Check sheet for the modelled part. Datum: model origin and axes. Units: mm. Face numbers are marked on the shaded views. A direction names the side the tool comes from. Give positions to 0.01 mm unless a question says otherwise; leave off trailing zeros. Order: outer loops, then holes, each group sorted by start corner. A loop starts at its lowest first (then second) coordinate and runs counter-clockwise, first axis right, second up.
from build123d import *

# Parameters (mm, degrees)
SKETCH_1_R      = 3.5
SKETCH_1_R_2    = 1.4
EXTRUDE_1_DEPTH = 2


with BuildPart() as part:
    # 草图1 → 凸台-拉伸1 (new body)
    with BuildSketch(Plane.XY):
        with BuildLine():
            Line((-10, -2), (-6.34428877, -2))
            ThreePointArc((-6.34428877, -2), (-5.378196987, -2.248809928), (-4.652478431, -2.933333333))
            ThreePointArc((-4.652478431, -2.933333333), (0, -5.5), (4.652478431, -2.933333333))
            ThreePointArc((4.652478431, -2.933333333), (5.378196987, -2.248809928), (6.34428877, -2))
            Line((6.34428877, -2), (10, -2))
            Line((10, -2), (10, 2))
            Line((10, 2), (6.34428877, 2))
            ThreePointArc((6.34428877, 2), (5.378196987, 2.248809928), (4.652478431, 2.933333333))
            ThreePointArc((4.652478431, 2.933333333), (0, 5.5), (-4.652478431, 2.933333333))
            ThreePointArc((-4.652478431, 2.933333333), (-5.378196987, 2.248809928), (-6.34428877, 2))
            Line((-6.34428877, 2), (-10, 2))
            Line((-10, 2), (-10, -2))
        make_face()
        Circle(SKETCH_1_R, mode=Mode.SUBTRACT)
        with Locations((-7.5, 0)):
            Circle(SKETCH_1_R_2, mode=Mode.SUBTRACT)
        with Locations((7.5, 0)):
            Circle(SKETCH_1_R_2, mode=Mode.SUBTRACT)
    extrude(amount=EXTRUDE_1_DEPTH)


solid = part.part
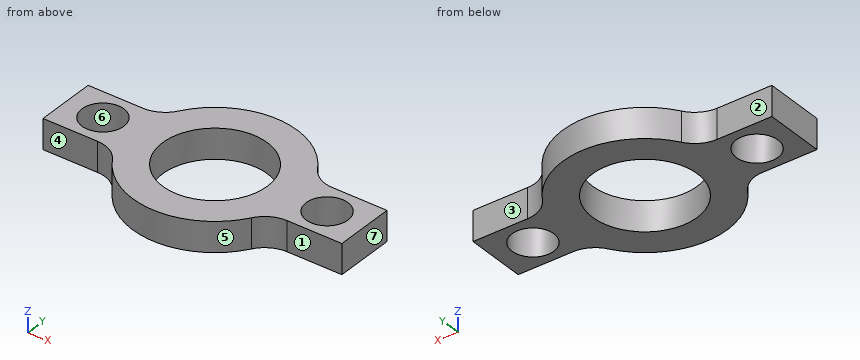
1) Draft check along X on the marked faces 5, 6 and 7. Enter one of: +X half, -X half, draft (parallel to the pull), parting line (faces both ways), or undercut.
Recorded:
face 5: parting line
face 6: undercut
face 7: +X half
2) Section check A-A, the plane y = 0. Record the cut outline in (x, z), then the cut area to 3 significant figures.
Recorded:
outline: (-10, 0) - (-8.9, 0) - (-8.9, 2) - (-10, 2) - close; (-6.1, 0) - (-3.5, 0) - (-3.5, 2) - (-6.1, 2) - close; (3.5, 0) - (6.1, 0) - (6.1, 2) - (3.5, 2) - close; (8.9, 0) - (10, 0) - (10, 2) - (8.9, 2) - close
area: 14.8 mm2
3) Section check C-C, the plane z = 1.45. Record the cut outline in (x, y), then the cut area to 3 significant figures.
Recorded:
outline: (-10, -2) - (-6.34, -2) arc R2 cw to (-4.65, -2.93) arc R5.5 ccw to (4.65, -2.93) arc R2 cw to (6.34, -2) - (10, -2) - (10, 2) - (6.34, 2) arc R2 cw to (4.65, 2.93) arc R5.5 ccw to (-4.65, 2.93) arc R2 cw to (-6.34, 2) - (-10, 2) - close; hole circle Ø2.8 at (-7.5, 0); hole circle Ø7 at (0, 0); hole circle Ø2.8 at (7.5, 0)
area: 82.1 mm2
4) Set-up check for the marked faces 1, 2, 3 and 4: record each of +Z, -Z, +X, -X, +Y, -Y from which the full face is reachable in a straight line by a thin tool's end or side.
Recorded:
face 1: +Z, -Z, +X, -Y
face 2: +Z, -Z, -X, +Y
face 3: +Z, -Z, +X, +Y
face 4: +Z, -Z, -X, -Y
5) Depth check by flat-ended pin: pin 1 Ø2 at (x, y) = (7.5, 0) entering from +Z; pin 2 Ø0.6 at (x, z) = (9, 1) entering from +Y. Enter the tip coordinate at first touch or a pass-through.
Recorded:
pin 1: passes through
pin 2: stops at y = 2
6) Section check D-D, the plane x = -7.5. Record the cut outline in (y, z), then the cut area to 3 significant figures.
Recorded:
outline: (-2, 0) - (-1.4, 0) - (-1.4, 2) - (-2, 2) - close; (1.4, 0) - (2, 0) - (2, 2) - (1.4, 2) - close
area: 2.40 mm2
7) Section check B-B, the plane x = 0. Record the cut outline in (y, z), then the cut area to 3 significant figures.
Recorded:
outline: (-5.5, 0) - (-3.5, 0) - (-3.5, 2) - (-5.5, 2) - close; (3.5, 0) - (5.5, 0) - (5.5, 2) - (3.5, 2) - close
area: 8.00 mm2
8) Material ranges on L1, parallel to Y at x = -7.5, z = 0.9; L2, parallel to X at y = 0.5, z = 0.1; L3, parallel to Y at x = 8, z = 0.4, recorded low to high.
Recorded:
L1: y = -2 to -1.4, 1.4 to 2
L2: x = -10 to -8.81, -6.19 to -3.46, 3.46 to 6.19, 8.81 to 10
L3: y = -2 to -1.31, 1.31 to 2
